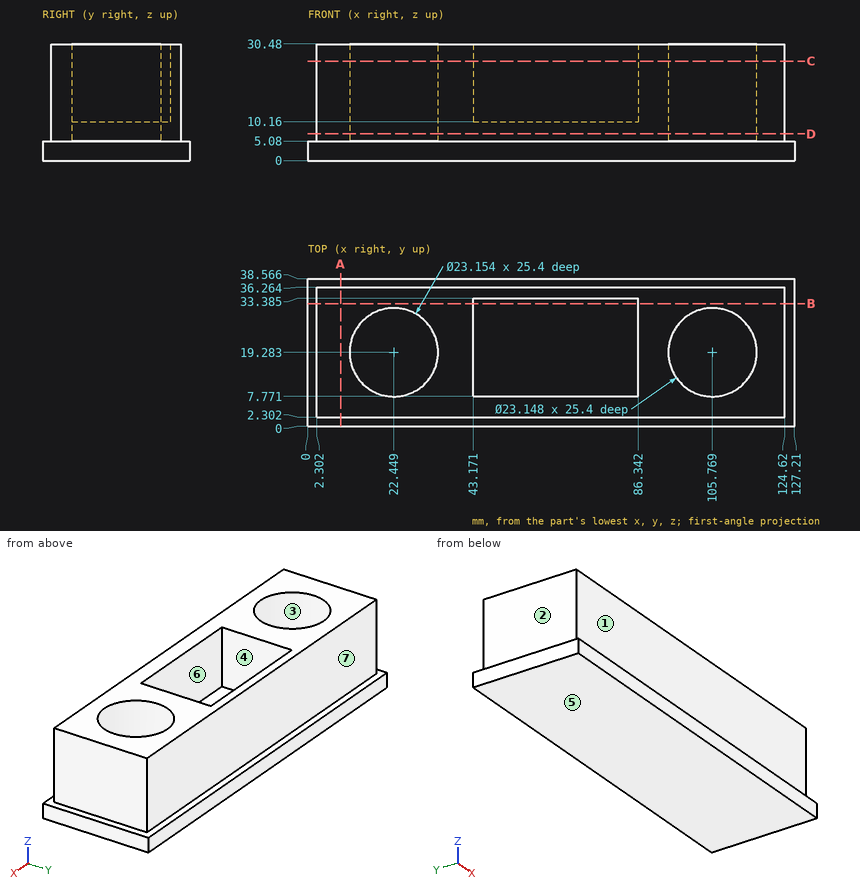
Check sheet for the drawn part. Datum: minimum x, y, z corner. Units: mm. A direction names the side the tool comes from. Round coordinates to 2 decimals unless told otherwise and drop trailing zeros. Order: outer loops, then holes, each group sorted by start corner. A loop starts at its lowest first (then second) coordinate and runs counter-clockwise, first axis right, second up. Notation, with made-up numbers: M 28,77.5 L 37,77.5 A17 ccw 37,103.5 Z; hole C 7,52 d2. An arc over 180 degrees is marked long. Write each question's results on one line, items separated by ' | '. Start each with the question number.
1. Go/stop test with flat-tipped pins: P1, Ø10, axis at y = 20.5, z = 19, coming from the +X side; P2, Ø10, axis at x = 61.5, z = 16, coming from the +Y side; P3, Ø10, axis at x = 62, z = 20.5, coming from the -Y side. Record where each tip stops, or that it passes through.
2. Draft check along Y on the marked faces 4, 5, 6 and 7. Enter one of: pulls with the +Y half, pulls with the -Y half, needs draft (parallel to the pull), parting line crosses it, or undercut.
3. Cross-section at A-A on x = 8.5. Record the boundary of the cut face in (y, z).
4. Cross-section at B-B on y = 32. Record the boundary of the cut face in (x, z).
5. Cross-section at D-D on z = 7. Record the boundary of the cut face in (x, y) (1 decimal).
6. Set-up check for the marked faces 1, 2 and 3: record each of +Z, -Z, +X, -X, +Y, -Y from which the full face is reachable in a straight line by a thin tool's end or side.
7. Material ranges on L1, parallel to Y at x = 74.5, z = 12 (1 decimal); L2, parallel to X at y = 10, z = 29 (1 decimal); L3, parallel to X at y = 21, z = 29 (1 decimal), recorded low to high. Write a range as from..to.
8. Cross-section at C-C on z = 26. Record the boundary of the cut face in (x, y) (1 decimal).
Resolved:
1) P1: x = 124.62 | P2: y = 36.26 | P3: y = 2.3
2) face 4: undercut | face 5: needs draft | face 6: undercut | face 7: pulls with the +Y half
3) outline: M 0,0 L 38.57,0 L 38.57,5.08 L 36.26,5.08 L 36.26,30.48 L 2.3,30.48 L 2.3,5.08 L 0,5.08 Z
4) outline: M 0,0 L 127.21,0 L 127.21,5.08 L 124.62,5.08 L 124.62,30.48 L 86.34,30.48 L 86.34,10.16 L 43.17,10.16 L 43.17,30.48 L 2.3,30.48 L 2.3,5.08 L 0,5.08 Z
5) outline: M 2.3,2.3 L 124.6,2.3 L 124.6,36.3 L 2.3,36.3 Z; hole C 22.4,19.3 d23.2; hole C 105.8,19.3 d23.1
6) face 1: +Z, +X, -X, -Y | face 2: +Z, -X, +Y, -Y | face 3: +Z
7) L1: 2.3..7.8, 33.4..36.3 | L2: 2.3..15.5, 29.4..43.2, 86.3..98.9, 112.7..124.6 | L3: 2.3..11, 33.9..43.2, 86.3..94.3, 117.2..124.6
8) outline: M 2.3,2.3 L 124.6,2.3 L 124.6,36.3 L 2.3,36.3 Z; hole C 22.4,19.3 d23.2; hole M 43.2,7.8 L 86.3,7.8 L 86.3,33.4 L 43.2,33.4 Z; hole C 105.8,19.3 d23.1
